```python
from build123d import *

# Parameters (mm, degrees)
F0_R     = 6.975
F0_R_2   = 6.05
F1_DEPTH = 38
F3_R     = 3.25
F4_DEPTH = 14


with BuildPart() as f1:
    # F0 (on Right) → F1 (new body)
    with BuildSketch(Plane.YZ):
        Circle(F0_R)
        Circle(F0_R_2, mode=Mode.SUBTRACT)
    extrude(amount=F1_DEPTH)

    # F3 (on offset) → F4 (cut)
    with BuildSketch(Plane.XY.offset(7)):
        with Locations((12, 0)):
            Circle(F3_R)
        with Locations((26, 0)):
            Circle(F3_R)
    extrude(amount=-F4_DEPTH, mode=Mode.SUBTRACT)


solid = f1.part
```
The model under review builds one solid part; all positions refer to its coordinate system, in mm. Coordinates: 2 decimals unless noted, no trailing zeros. Loops run counter-clockwise (first coordinate to the right, second up) from the corner with the lowest first, then second, coordinate; pieces in that order, holes last. Notation, with made-up numbers: (-13.5, 48.5) -> (27.5, 48.5) arc R28 ccw to (27.5, 75.5) -> close; hole circle Ø5 at (41, 25). An arc over 180 degrees is marked (long way). Answer as CSV lines item,"result".
Item 1: Take a section at B-B, the plane y = 0. State the section outline as (x, z) points (3 decimals).
Results below:
outline,"(0, -6.975) -> (8.75, -6.975) -> (8.75, -6.05) -> (0, -6.05) -> close; (0, 6.05) -> (8.75, 6.05) -> (8.75, 6.975) -> (0, 6.975) -> close; (15.25, -6.975) -> (22.75, -6.975) -> (22.75, -6.05) -> (15.25, -6.05) -> close; (15.25, 6.05) -> (22.75, 6.05) -> (22.75, 6.975) -> (15.25, 6.975) -> close; (29.25, -6.975) -> (38, -6.975) -> (38, -6.05) -> (29.25, -6.05) -> close; (29.25, 6.05) -> (38, 6.05) -> (38, 6.975) -> (29.25, 6.975) -> close"
Item 2: For L1, parallel to X at y = 0, z = 6.3; L2, parallel to Y at x = 30, z = 2.5; L3, parallel to Z at x = 19, y = 0 (3 decimals), list the stretches that pass through material, from the lowest coordinate up.
Results below:
L1,"x = 0 to 8.75, 15.25 to 22.75, 29.25 to 38"
L2,"y = -6.51 to -5.51, 5.51 to 6.51"
L3,"z = -6.975 to -6.05, 6.05 to 6.975"
Item 3: Take a section at C-C, the plane x = 13. State the section outline as (y, z) points (3 decimals), and give its area (3 significant figures).
Results below:
outline,"(-3.092, -6.252) -> (-3.092, -5.2) arc R6.05 cw to (-3.092, 5.2) -> (-3.092, 6.252) arc R6.975 ccw to start; (3.092, -6.252) arc R6.975 ccw to (3.092, 6.252) -> (3.092, 5.2) arc R6.05 cw to (3.092, -5.2) -> close"
area,"25.9 mm2"
Item 4: Take a section at D-D, the plane x = 20.5. State the section outline as (y, z) points (3 decimals), and give its area (3 significant figures).
Results below:
outline,"circle Ø13.95 at (0, 0); hole circle Ø12.1 at (0, 0)"
area,"37.9 mm2"
Item 5: Draft analysis for pull direction X (two halves, no side actions). For faces 1 (the flat face through (0, -2, 6)), 2 (the cylindrical face through (29.002, -1.245, -6.237)), 3 (the flat face through (38, -2, 6)), state which applies: +X half, -X half, draft (parallel to the pull), parting line (faces both ways), or undercut.
Results below:
face 1,"-X half"
face 2,"undercut"
face 3,"+X half"
Item 6: Take a section at A-A, the plane z = 0. State the section outline as (x, y) points (3 decimals), and give its area (3 significant figures).
Results below:
outline,"(0, -6.975) -> (38, -6.975) -> (38, -6.05) -> (0, -6.05) -> close; (0, 6.05) -> (38, 6.05) -> (38, 6.975) -> (0, 6.975) -> close"
area,"70.3 mm2"
Item 7: Insertion check: pin 1 (5 mm diameter, centred on x = 8, z = 0.5, fed in from +Y) (3 decimals); pin 2 (2 mm diameter, centred on x = 12.5, z = -3.5, fed in from -Y); pin 3 (6 mm diameter, centred on y = 0.5, z = -1, fed in from -X); pin 4 (2 mm diameter, centred on x = 27, z = 3.5, fed in from +Y). Each pin has a flat end and moves straight along its axis. Give the tip position at first contact, or say it passes through.
Results below:
pin 1,"stops at y = 6.975"
pin 2,"stops at y = -6.51"
pin 3,"passes through"
pin 4,"stops at y = 6.51"
